Build history of the part. All positions in model axes, mm. A direction names the side the tool comes from. Give positions to 0.01 mm unless a question says otherwise; leave off trailing zeros. Write each loop counter-clockwise with the first axis right and the second up, starting at its lowest first coordinate (ties: lowest second). Pieces come first, ordered by that corner, then holes. Notation, with made-up numbers: M -25,88 L 9,88 A32 cw 9,120 Z; hole C 16.5,27.25 d8. An arc over 180 degrees is marked long. Return JSON: item names as keys, results as strings. Group by question number.
Q1. Band-saw the part on A-A, the plane y = 2. Give the cut face in (x, z) (3 decimals), then the cut area to 3 significant figures.
Q2. Band-saw the part on B-B, the plane x = 11.5. Give the cut face in (y, z) (3 decimals), then the cut area to 3 significant figures.
Q3. Band-saw the part on D-D, the plane z = 35.5. Give the cut face in (x, y).
Q4. Band-saw the part on C-C, the plane z = 49. Give the cut face in (x, y).
Q5. Pull direction X, two halves, no side cores. Call faces 3 (the flat face through (53.55, -0.07, 23.34)), 4 (the cylindrical face through (40.493, -18.805, 49.324)), 5 (the flat face through (56, 4.762, 33)): +X half, -X half, draft (parallel to the pull), parting line (faces both ways), or undercut.
Q6. Wall check: probe 1 along Y at (x, z) = (12, 50); probe 2 along X at (y, z) = (-14, 30); probe 3 along Z at (x, y) = (42, -10.5) (3 decimals). Give the ranges that are in metal, low to high.
Q7. Flat gauge pins, fed straight in: pin 1 Ø10 at (x, y) = (35.5, -8.5) entering from -Z; pin 2 Ø6 at (x, y) = (73, -7.5) entering from -Z; pin 3 Ø14.5 at (x, y) = (46.05, -19.05) entering from -Z (3 decimals); pin 4 Ø9 at (x, y) = (12.7, 0) entering from +Z. Where does each tip first touch, or does it go through?
Q8. Tool access for faces 1 (the cylindrical face through (41.636, 15.665, 49.324)), 2 (the flat face through (36, 7, 41.275)): list every direction of +Z, -Z, +X, -X, +Y, -Y with a clear straight run to the whole face (end or side of a thin tool).
from build123d import *

# Parameters (mm, degrees)
F0_R     = 19.05
F1_DEPTH = 31.75
F2_DEPTH = 4.7625
F4_DEPTH = 57.151
F3_R     = 5.5626
F5_DEPTH = 57.151


with BuildPart() as f1:
    # F0 (on Front) → F1 (new body, symmetric)
    with BuildSketch(Plane.XZ):
        with BuildLine():
            Line((96.8502, 57.15), (0, 57.15))
            Line((0, 57.15), (0, 41.275))
            Line((0, 41.275), (27.0002, 41.275))
            Line((27.0002, 41.275), (58.8827221407, 41.275))
            ThreePointArc((58.8827221407, 41.275), (65.8929323283, 38.1984554837), (68.3745916055, 30.95625))
            ThreePointArc((68.3745916055, 30.95625), (71.0782767463, 16.2324477191), (80.8551747025, 4.8961108636))
            ThreePointArc((80.8551747025, 4.8961108636), (124.1737693319, 20.2111979959), (96.8502, 57.15))
        make_face()
        with Locations((96.8502, 28.575)):
            Circle(F0_R, mode=Mode.SUBTRACT)
    extrude(amount=F1_DEPTH, both=True)

    # F0 (on Front) → F2 (join, symmetric)
    with BuildSketch(Plane.XZ):
        with BuildLine():
            Line((27.0002, 41.275), (80.8551747025, 4.8961108636))
            ThreePointArc((80.8551747025, 4.8961108636), (71.0782767463, 16.2324477191), (68.3745916055, 30.95625))
            ThreePointArc((68.3745916055, 30.95625), (65.8929323283, 38.1984554837), (58.8827221407, 41.275))
            Line((58.8827221407, 41.275), (27.0002, 41.275))
        make_face()
    extrude(amount=F2_DEPTH, both=True)

    # F3 (on face) → F4 (cut, through all)
    with BuildSketch(Plane.XY.offset(57.15)):
        with BuildLine():
            ThreePointArc((0, 1.86e-08), (1.7161647423, 6.3753715996), (6.4008445559, 11.0277214642))
            Line((6.4008445559, 11.0277214642), (39.7510445559, 30.0777214642))
            ThreePointArc((39.7510445559, 30.0777214642), (42.7915240875, 31.3248128824), (46.0502, 31.75))
            Line((46.0502, 31.75), (0, 31.75))
            Line((0, 31.75), (0, 1.86e-08))
        make_face()
        with BuildLine():
            ThreePointArc((6.4008445559, -11.0277214642), (1.716164733, -6.3753715835), (0, 1.86e-08))
            Line((0, 1.86e-08), (0, -31.75))
            Line((0, -31.75), (46.0502, -31.75))
            ThreePointArc((46.0502, -31.75), (42.7915240875, -31.3248128824), (39.7510445559, -30.0777214642))
            Line((39.7510445559, -30.0777214642), (6.4008445559, -11.0277214642))
        make_face()
    extrude(amount=-F4_DEPTH, mode=Mode.SUBTRACT)

    # F3 (on face) → F5 (cut, through all)
    with BuildSketch(Plane.XY.offset(57.15)):
        with Locations((12.7, 0)):
            Circle(F3_R)
        with Locations((46.0502, 19.05)):
            Circle(F3_R)
        with Locations((46.0502, -19.05)):
            Circle(F3_R)
    extrude(amount=-F5_DEPTH, mode=Mode.SUBTRACT)


solid = f1.part
From the geometry:
{
 "1": {"outline": "M 0.158,41.275 L 7.509,41.275 L 7.509,57.15 L 0.158,57.15 Z; M 17.891,41.275 L 27,41.275 L 80.855,4.896 A28.575 ccw long 96.85,57.15 L 17.891,57.15 Z; hole C 96.85,28.575 d38.1", "area": "3,130 mm^2"},
 "2": {"outline": "M -13.94,41.275 L -5.432,41.275 L -5.432,57.15 L -13.94,57.15 Z; M 5.432,41.275 L 13.94,41.275 L 13.94,57.15 L 5.432,57.15 Z", "area": "270 mm^2"},
 "3": {"outline": "M 35.55,-4.76 L 67.64,-4.76 L 67.64,-31.75 L 79.1,-31.75 L 79.1,31.75 L 67.64,31.75 L 67.64,4.76 L 35.55,4.76 Z; M 114.6,-31.75 L 124.57,-31.75 L 124.57,31.75 L 114.6,31.75 Z"},
 "4": {"outline": "M 6.4,-11.03 L 39.75,-30.08 A12.7 ccw 46.05,-31.75 L 116.83,-31.75 L 116.83,31.75 L 46.05,31.75 A12.7 ccw 39.75,30.08 L 6.4,11.03 A12.7 ccw Z; hole C 12.7,0 d11.13; hole C 46.05,-19.05 d11.13; hole C 46.05,19.05 d11.13"},
 "5": {"face 3": "-X half", "face 4": "undercut", "face 5": "draft"},
 "6": {"probe 1": "y = -14.23 to -5.52, 5.52 to 14.23", "probe 2": "x = 68.31 to 77.85, 115.85 to 125.39", "probe 3": "z = 41.275 to 57.15"},
 "7": {"pin 1": "stops at z = 33.29", "pin 2": "stops at z = 9.04", "pin 3": "stops at z = 41.275", "pin 4": "passes through"},
 "8": {"face 1": "+Z, -Z", "face 2": "-Z, -X"}
}
